from build123d import *

# Parameters (mm, degrees)
SKETCH2_W          = 19
SKETCH2_H          = 15.9
SKETCH2_W_2        = 15
SKETCH2_H_2        = 11.9
CUT_EXTRUDE1_DEPTH = 2.9


with BuildPart() as part:
    # Sketch1 → Revolve1 (revolve)
    with BuildSketch(Plane(origin=(0, 0, 0), x_dir=(1, 0, 0), z_dir=(0, 1, 0))):
        Polygon((-50.15, 0.75), (-50.15, 1.95), (-43.05, 2.322095233), (-43.05, 4.1), (-46.55, 4.1), (-46.55, 4.74), (-39.7, 4.74), (-39.7, 5), (-32.85, 5), (-32.85, 4.5), (47.25, 4.5), (47.25, 6.9), (50.15, 6.9), (50.15, 2.3), (-32.85, 2.3), (-32.85, 0.75), align=None)
    revolve(axis=Axis((50.15, 0, 0), (-1, 0, 0)))

    # Sketch2 → Cut-Extrude1 (cut)
    with BuildSketch(Plane(origin=(50.15, 0, 0), x_dir=(0, 0, -1), z_dir=(1, 0, 0))):
        Rectangle(SKETCH2_W, SKETCH2_H)
        Rectangle(SKETCH2_W_2, SKETCH2_H_2, mode=Mode.SUBTRACT)
    extrude(amount=-CUT_EXTRUDE1_DEPTH, mode=Mode.SUBTRACT)


solid = part.part
CAD build for the part. Positions are in the model's coordinates, mm. A direction names the side the tool comes from. Round coordinates to 2 decimals unless told otherwise and drop trailing zeros. Loops run counter-clockwise (first coordinate to the right, second up) from the corner with the lowest first, then second, coordinate; pieces in that order, holes last.
(1) Cut at A-A (x = 25.5). Give the cut face in (y, z).
(2) Drop flat-ended pins along their axis: pin 1 (1.7 mm diameter, centred on y = 0, z = 0, fed in from -X); pin 2 (1.5 mm diameter, centred on x = 2.5, z = -3, fed in from -Y); pin 3 (2 mm diameter, centred on x = -20, z = -4, fed in from -Y); pin 4 (5 mm diameter, centred on x = -27, y = 4.5, fed in from +Z). Give the stop position or say it passes through.
(3) Which spindle directions (+Z, -Z, +X, -X, +Y, -Y) get a long thin tool onto all of the face, cutting with end or side? Do faces 1 (the cylindrical face through (-36.23, 4.88, 1.08)), 2 (the flat face through (49, 5.95, 0)), 3 (the flat face through (-32.85, -1, 1)). Say none if no direction does.
(4) Wall check: line 1 along Y through (x, z) = (-37.25, 0); line 2 along Y through (x, z) = (-43.8, 0); line 3 along Z through (x, y) = (-43.95, 0). Give the ranges that are in metal, low to high.
(5) Two-plate mould, pull along Y, no slides. Class faces 4 (the cylindrical face through (8.069, 1.4, 1.825)), 5 (the cylindrical face through (7.76, -4.46, 0.59)), 6 (the flat face through (47.25, 0, 5)), 7 (the cylindrical face through (-44.824, -4.065, 0.534)): +Y half, -Y half, draft (parallel to the pull), parting line (faces both ways), or undercut.
Findings below:
1. outline: circle Ø9 at (0, 0); hole circle Ø4.6 at (0, 0)
2. pin 1: stops at x = -50.15
2. pin 2: stops at y = -3.9
2. pin 3: stops at y = -3.35
2. pin 4: stops at z = 4.03
3. face 1: -X
3. face 2: +Z, -Z, +X, -X, +Y
3. face 3: +X
4. line 1: y = -5 to -0.75, 0.75 to 5
4. line 2: y = -4.74 to -4.1, -2.28 to -0.75, 0.75 to 2.28, 4.1 to 4.74
4. line 3: z = -4.74 to -4.1, -2.27 to -0.75, 0.75 to 2.27, 4.1 to 4.74
5. face 4: undercut
5. face 5: parting line
5. face 6: draft
5. face 7: undercut
